Input: part model. Units: mm. Frame: model coordinates. A direction names the side the tool comes from. Round coordinates to 2 decimals unless told otherwise and drop trailing zeros. Loops run counter-clockwise (first coordinate to the right, second up) from the corner with the lowest first, then second, coordinate; pieces in that order, holes last. Notation, with made-up numbers: (0.5, 47) - (54.5, 47) arc R34 ccw to (54.5, 81) - close; hole circle Ø7 at (62.5, 41.5). An arc over 180 degrees is marked (long way). One line per question, with ' | ' between items. Start each with the question number.
Item 1: Section B-B, the plane y = -16.5. Return loops of the section in (x, z), plus the area to 3 significant figures.
Item 2: Section A-A, the plane z = -8.25. Return loops of the section in (x, y).
Item 3: Draft query along X for faces 1 (the face through (59.885, -9.7, -0.136)), 2 (the face through (39, -12, -9.71)), 3 (the face through (64, 0, 9.71)). Return one class per face: pulls with the +X half, pulls with the -X half, needs draft (parallel to the pull), parting line crosses it, or undercut.
Item 4: Set-up query: faces 4 (the face through (60.441, 9.976, -0.136)), 5 (the face through (39, 20, 0)), 6 (the face through (39, -12, 9.71)). Return all of +Z, -Z, +X, -X, +Y, -Y with unobstructed straight access to the full face (end or side cutting, diameter ignored); none if empty.
Item 5: First-contact query: pin 1 (6 mm diameter, centred on y = 9, z = 1.5, fed in from +X); pin 2 (12 mm diameter, centred on y = -7.5, z = 2, fed in from +X). Flat tips, straight axial feed; report the tip coordinate or a pass-through.
Item 6: Section C-C, the plane x = 43. Return loops of the section in (y, z).
Item 7: Material intervals for line 1 along Z through (x, y) = (62, 12.5); line 2 along X through (y, z) = (14, -5.5); line 3 along X through (y, z) = (12, 4), sorted ascending.
```python
from build123d import *

# Parameters (mm, degrees)
F0_W     = 40
F0_H     = 20
F2_DEPTH = 80
F3_T     = -0.29
F5_DEPTH = 20


with BuildPart() as f2:
    # F0 (on Right) → F2 (new body)
    with BuildSketch(Plane.YZ):
        Rectangle(F0_W, F0_H)
    extrude(amount=F2_DEPTH)

    # F3
    f3_openings = [f2.faces().sort_by_distance(p)[0] for p in [
        (80, 0, 0),
    ]]
    offset(amount=F3_T, openings=f3_openings)

    # F4 (on face) → F5 (join)
    with BuildSketch(Plane(origin=(0, 0, -10), x_dir=(1, 0, 0), z_dir=(0, 0, -1))):
        Polygon((39.6736521938, 0), (40, -0.1618533906), (40.3263478062, 0), (40, 0.1618533906), align=None)
        Polygon((40, 0.1618533906), (40.3263478062, 0), (80, 19.6762932188), (80, 20), align=None)
        Polygon((0, -19.6762932188), (0, -20), (40, -0.1618533906), (39.6736521938, 0), align=None)
        Polygon((0, 19.6762932188), (39.6736521938, 0), (40, 0.1618533906), (0, 20), align=None)
        Polygon((40.3263478062, 0), (40, -0.1618533906), (80, -20), (80, -19.6762932188), align=None)
    extrude(amount=-F5_DEPTH)


solid = f2.part
```
Return value:
1) outline: (0, -10) - (80, -10) - (80, -9.71) - (73.6, -9.71) - (73.6, 9.71) - (80, 9.71) - (80, 10) - (0, 10) - close; hole (0.29, -9.71) - (6.4, -9.71) - (6.4, 9.71) - (0.29, 9.71) - close; hole (7.06, -9.71) - (72.94, -9.71) - (72.94, 9.71) - (7.06, 9.71) - close | area: 77.4 mm2
2) outline: (0, -20) - (80, -20) - (80, -19.68) - (40.33, 0) - (80, 19.68) - (80, 20) - (0, 20) - close; hole (0.29, -19.53) - (39.67, 0) - (0.29, 19.53) - close; hole (0.58, -19.71) - (79.42, -19.71) - (40, -0.16) - close; hole (0.58, 19.71) - (40, 0.16) - (79.42, 19.71) - close
3) face 1: pulls with the +X half | face 2: undercut | face 3: needs draft
4) face 4: +X | face 5: +Z, -Z, +X, -X, +Y | face 6: none
5) pin 1: x = 64.52 | pin 2: x = 67.55
6) outline: (-20, -10) - (20, -10) - (20, 10) - (-20, 10) - close; hole (-19.71, -9.71) - (-1.65, -9.71) - (-1.65, 9.71) - (-19.71, 9.71) - close; hole (-1.33, -9.71) - (1.33, -9.71) - (1.33, 9.71) - (-1.33, 9.71) - close; hole (1.65, -9.71) - (19.71, -9.71) - (19.71, 9.71) - (1.65, 9.71) - close
7) line 1: -10 to -9.71, 9.71 to 10 | line 2: 0 to 0.29, 11.45 to 12.1, 67.9 to 68.55 | line 3: 0 to 0.29, 15.48 to 16.13, 63.87 to 64.52
